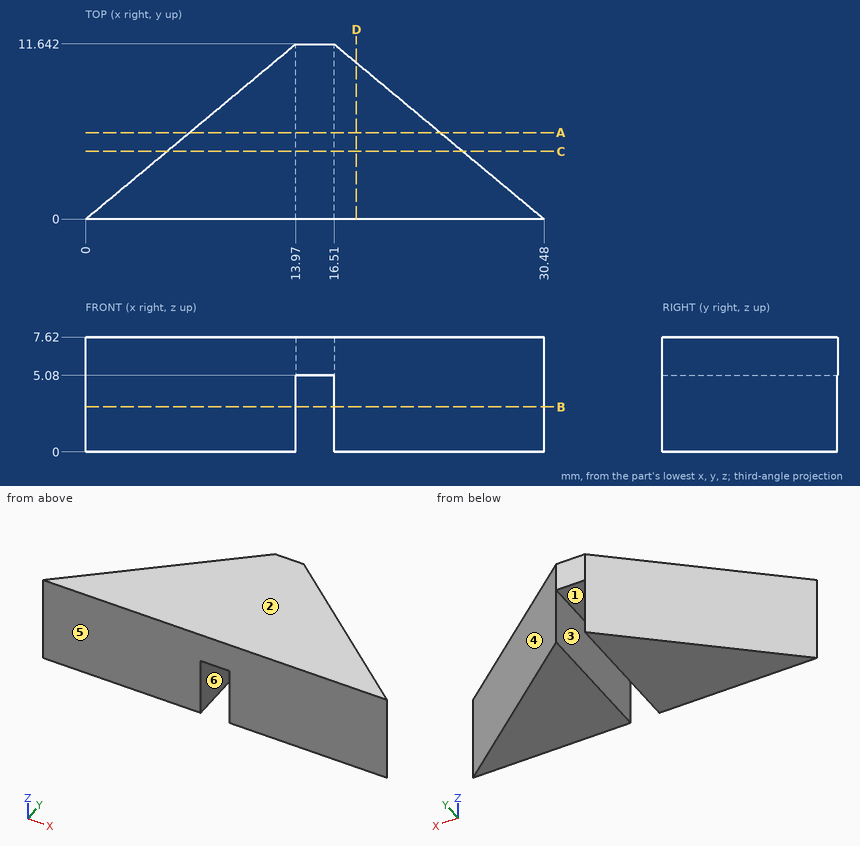
For this review, use the dimensioned drawing (mm, ordinates from the lowest corner) and the shaded views. A direction names the side the tool comes from. Round coordinates to 2 decimals unless told otherwise and drop trailing zeros. Order: outer loops, then holes, each group sorted by start corner. A loop starts at its lowest first (then second) coordinate and runs counter-clockwise, first axis right, second up. Notation, with made-up numbers: (31, 66.25) -> (52, 66.25) arc R28 cw to (52, 100.25) -> close; hole circle Ø4 at (71, 50.5). An arc over 180 degrees is marked (long way). Use CSV: the item, a comma, the result in double quotes. Start each with the question number.
(1) Consider section B-B on z = 3. Write out the cut boundary in (x, y), and give its area (3 significant figures).
(2) Tool access review of the marked faces 1 and 2: name each direction out of +Z, -Z, +X, -X, +Y, -Y from which nothing blocks a thin tool from reaching the whole face with its end or side.
(3) Mouldability with a two-part tool opening along X and no side actions: class the marked faces 3, 4, 5 and 6 as pulls with the +X half, pulls with the -X half, needs draft (parallel to the pull), parting line crosses it, or undercut.
(4) Wall thickness on probe 1 along Z at (x, y) = (15, 10); probe 2 along X at (y, z) = (7, 2.75); probe 3 along X at (y, z) = (5, 3.5): over which ranges is each line inside the solid? List them lowest first. Write a range as from..to.
(5) Consider section A-A on y = 5.75. Write out the cut boundary in (x, z), and give its area (3 significant figures).
(6) Consider section C-C on y = 4.5. Write out the cut boundary in (x, z), and give its area (3 significant figures).
(7) Insertion check: pin 1 (2 mm diameter, centred on y = 2.5, z = 5.5, fed in from +X); pin 2 (1 mm diameter, centred on x = 15, z = 3, fed in from -Y); pin 3 (0.8 mm diameter, centred on x = 15, y = 4, fed in from -Z); pin 4 (1.5 mm diameter, centred on y = 5.5, z = 3.5, fed in from +X). Each pin has a flat end and moves straight along its axis. Give the tip position at first contact, or say it passes through.
(8) Consider section D-D on x = 18. Write out the cut boundary in (y, z).
Responses:
1,outline,"(0, 0) -> (13.97, 0) -> (13.97, 11.64) -> close; (16.51, 0) -> (30.48, 0) -> (16.51, 11.64) -> close"
1,area,"163 mm²"
2,face 1,"-Z, +Y, -Y"
2,face 2,"+Z, +X, -X, +Y, -Y"
3,face 3,"undercut"
3,face 4,"pulls with the +X half"
3,face 5,"needs draft"
3,face 6,"undercut"
4,probe 1,"5.08..7.62"
4,probe 2,"8.4..13.97, 16.51..22.08"
4,probe 3,"6..13.97, 16.51..24.48"
5,outline,"(6.9, 0) -> (13.97, 0) -> (13.97, 5.08) -> (16.51, 5.08) -> (16.51, 0) -> (23.58, 0) -> (23.58, 7.62) -> (6.9, 7.62) -> close"
5,area,"114 mm²"
6,outline,"(5.4, 0) -> (13.97, 0) -> (13.97, 5.08) -> (16.51, 5.08) -> (16.51, 0) -> (25.08, 0) -> (25.08, 7.62) -> (5.4, 7.62) -> close"
6,area,"137 mm²"
7,pin 1,"x = 28.68"
7,pin 2,"through"
7,pin 3,"z = 5.08"
7,pin 4,"x = 24.78"
8,outline,"(0, 0) -> (10.4, 0) -> (10.4, 7.62) -> (0, 7.62) -> close"
